Check sheet for the modelled part. Datum: model origin and axes. Units: mm. Face numbers are marked on the shaded views. A direction names the side the tool comes from. Give positions to 0.01 mm unless a question says otherwise; leave off trailing zeros. Order: outer loops, then holes, each group sorted by start corner. A loop starts at its lowest first (then second) coordinate and runs counter-clockwise, first axis right, second up. Notation, with made-up numbers: (54.5, 21) -> (108.5, 21) arc R5 cw to (108.5, 27) -> close; hole circle Ø1 at (51, 18.5). An arc over 180 degrees is marked (long way). Write each question's results on one line, items separated by ' | '.
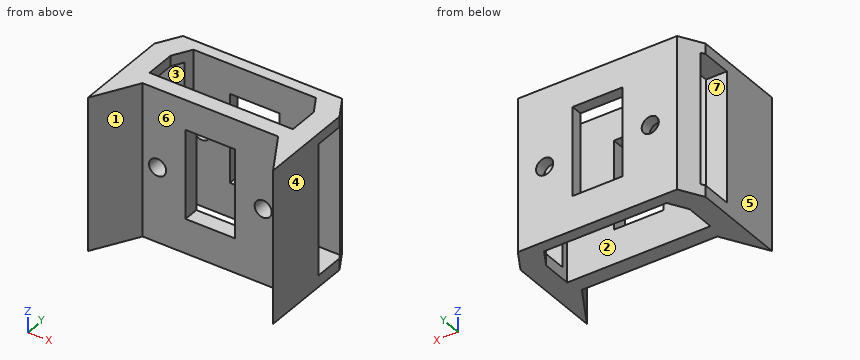
from build123d import *

# Parameters (mm, degrees)
PAD017_DEPTH       = 40
SKETCH041_W        = 13
SKETCH041_H        = 23.22
POCKET003014_DEPTH = 31.179264
POCKET003015_DEPTH = 40.001
SKETCH043_W        = 9.077184
SKETCH043_H        = 34.246025
POCKET003016_DEPTH = 49.253641
SKETCH050_R        = 2.24
POCKET003019_DEPTH = 31.179264


with BuildPart() as part:
    # Sketch040 → Pad017 (new body)
    with BuildSketch(Plane.XY):
        Polygon((-20.846346, 70.735185), (20.846346, 70.735185), (24.252641, 64.833161), (24.252641, 39.821736), (17.75, 51.08874), (-17.75, 51.08874), (-24.252641, 39.821736), (-24.252641, 64.833161), align=None)
    extrude(amount=PAD017_DEPTH)

    # Sketch041 → Pocket003014 (cut, through all)
    with BuildSketch(Plane.XZ.offset(-71)):
        with Locations((0, 20.61)):
            Rectangle(SKETCH041_W, SKETCH041_H)
    extrude(amount=POCKET003014_DEPTH, mode=Mode.SUBTRACT)

    # Sketch042 → Pocket003015 (cut, through all)
    with BuildSketch(Plane.XY.offset(40)):
        Polygon((-16.036429, 67.772269), (16.036429, 67.772269), (18.76456, 63.045287), (18.76456, 55.171417), (-18.76456, 55.171417), (-18.76456, 63.045287), align=None)
    extrude(amount=-POCKET003015_DEPTH, mode=Mode.SUBTRACT)

    # Sketch043 → Pocket003016 (cut, through all)
    with BuildSketch(Plane.YZ.offset(25)):
        with Locations((61.40538, 20.140725)):
            Rectangle(SKETCH043_W, SKETCH043_H)
    extrude(amount=-POCKET003016_DEPTH, mode=Mode.SUBTRACT)

    # Sketch050 → Pocket003019 (cut, through all)
    with BuildSketch(Plane.XZ.offset(-71)):
        with Locations((-13.83, 19.55)):
            Circle(SKETCH050_R)
        with Locations((13.83, 19.55)):
            Circle(SKETCH050_R)
    extrude(amount=POCKET003019_DEPTH, mode=Mode.SUBTRACT)


solid = part.part
1. Mould release check, pull along X, two halves, no side actions. Record for the marked faces 5, 6 and 7: +X half, -X half, draft (parallel to the pull), parting line (faces both ways), or undercut.
Verdict:
face 5: -X half | face 6: undercut | face 7: draft
2. Material ranges on probe 1 along X at (y, z) = (54.2, 19.55); probe 2 along Y at (x, z) = (13.5, 14); probe 3 along X at (y, z) = (69.15, 19.55), recorded low to high. Write a range as from..to.
Verdict:
probe 1: x = -24.25..-16.07, -11.59..-6.5, 6.5..11.59, 16.07..24.25 | probe 2: y = 51.09..55.17, 67.77..70.74 | probe 3: x = -21.76..-16.07, -11.59..-6.5, 6.5..11.59, 16.07..21.76
3. Section check A-A on x = 13.83. Record the cut outline in (y, z), then the cut area to 3 significant figures.
Verdict:
outline: (51.09, 0) -> (55.17, 0) -> (55.17, 17.31) -> (51.09, 17.31) -> close; (51.09, 21.79) -> (55.17, 21.79) -> (55.17, 40) -> (51.09, 40) -> close; (67.77, 0) -> (70.74, 0) -> (70.74, 17.31) -> (67.77, 17.31) -> close; (67.77, 21.79) -> (70.74, 21.79) -> (70.74, 40) -> (67.77, 40) -> close | area: 250 mm^2
4. Gauge pin test, flat ends, axial feed: pin 1 Ø18 at (x, z) = (-4.5, 14) entering from -Y; pin 2 Ø1 at (y, z) = (67.5, 34.5) entering from +X; pin 3 Ø1.5 at (y, z) = (70, 16.5) entering from +X; pin 4 Ø2.5 at (x, z) = (-13.83, 19.55) entering from -Y (3 decimals). Record the tip position at first contact, or that the pin passes through.
Verdict:
pin 1: stops at y = 51.09 | pin 2: stops at x = 23 | pin 3: stops at x = 21.7 | pin 4: passes through
5. Section check D-D on z = 5. Record the cut outline in (x, y), then the cut area to 3 significant figures.
Verdict:
outline: (-24.25, 39.82) -> (-17.75, 51.09) -> (17.75, 51.09) -> (24.25, 39.82) -> (24.25, 56.87) -> (18.76, 56.87) -> (18.76, 55.17) -> (-18.76, 55.17) -> (-18.76, 56.87) -> (-24.25, 56.87) -> close; (-23.61, 65.94) -> (-17.09, 65.94) -> (-16.04, 67.77) -> (16.04, 67.77) -> (17.09, 65.94) -> (23.61, 65.94) -> (20.85, 70.74) -> (-20.85, 70.74) -> close | area: 442 mm^2
6. Section check B-B on z = 14. Record the cut outline in (x, y).
Verdict:
outline: (-24.25, 39.82) -> (-17.75, 51.09) -> (-6.5, 51.09) -> (-6.5, 55.17) -> (-18.76, 55.17) -> (-18.76, 56.87) -> (-24.25, 56.87) -> close; (-23.61, 65.94) -> (-17.09, 65.94) -> (-16.04, 67.77) -> (-6.5, 67.77) -> (-6.5, 70.74) -> (-20.85, 70.74) -> close; (6.5, 51.09) -> (17.75, 51.09) -> (24.25, 39.82) -> (24.25, 56.87) -> (18.76, 56.87) -> (18.76, 55.17) -> (6.5, 55.17) -> close; (6.5, 67.77) -> (16.04, 67.77) -> (17.09, 65.94) -> (23.61, 65.94) -> (20.85, 70.74) -> (6.5, 70.74) -> close
7. Section check C-C on y = 60. Record the cut outline in (x, z), then the cut area to 3 significant figures.
Verdict:
outline: (-24.25, 0) -> (-18.76, 0) -> (-18.76, 3.02) -> (-24.25, 3.02) -> close; (-24.25, 37.26) -> (-18.76, 37.26) -> (-18.76, 40) -> (-24.25, 40) -> close; (18.76, 0) -> (24.25, 0) -> (24.25, 3.02) -> (18.76, 3.02) -> close; (18.76, 37.26) -> (24.25, 37.26) -> (24.25, 40) -> (18.76, 40) -> close | area: 63.2 mm^2
8. Access from +Z, -Z, +X, -X, +Y, -Y to the whole of each face (thin tool, end or side, straight path). Record for the marked faces 1, 2, 3 and 4.
Verdict:
face 1: +Z, -Z, -Y | face 2: +Z, -Z | face 3: +X, -X | face 4: +Z, -Z, +X, +Y, -Y
